from build123d import *
from OCP.BRepFilletAPI import BRepFilletAPI_MakeChamfer

# Parameters (mm, degrees)
BOSS_EXTRUDE1_DEPTH     = 15
SKETCH4_W               = 15
SKETCH4_H               = 15
BOSS_EXTRUDE2_DEPTH     = 9
CUT_EXTRUDE1_DEPTH      = 180.279015807
CUT_EXTRUDE1_DEPTH_BACK = 180.279015807
SKETCH2_R               = 2.2
SKETCH3_W               = 4.807860213
SKETCH3_H               = 184.008472667
CHAMFER1_SIZE           = 2.5
CHAMFER1_SIZE2          = 2.965251078
CHAMFER1_SIZE2_2        = 2.201823595
CHAMFER2_SIZE           = 2.5
BOSS_EXTRUDE5_DEPTH     = 3
BOSS_EXTRUDE3_DEPTH     = 2
BOSS_EXTRUDE6_DEPTH     = 2
FILLET2_R               = 1


with BuildPart() as part:
    # Sketch1 → Boss-Extrude1 (new body)
    with BuildSketch(Plane.XY):
        with BuildLine():
            Line((4.25, 16.976086121), (4.25, 10.145811944))
            ThreePointArc((4.25, 10.145811944), (0, -11), (-4.25, 10.145811944))
            Line((-4.25, 10.145811944), (-4.25, 16.976086121))
            ThreePointArc((-4.25, 16.976086121), (-12.969277239, 11.74937649), (-17.312062276, 2.557831066))
            Line((-17.312062276, 2.557831066), (-40, -151))
            Line((-40, -151), (-55, -151))
            Line((-55, -151), (-55, -160))
            Line((-55, -160), (55, -160))
            Line((55, -160), (55, -151))
            Line((55, -151), (40, -151))
            Line((40, -151), (17.312062276, 2.557831066))
            ThreePointArc((17.312062276, 2.557831066), (12.969277239, 11.74937649), (4.25, 16.976086121))
        make_face()
        Polygon((12.694157412, -17.5), (32.418580877, -151), (2.5, -151), (2.5, -17.5), align=None, mode=Mode.SUBTRACT)
        Polygon((-12.694157412, -17.5), (-2.5, -17.5), (-2.5, -151), (-32.418580877, -151), align=None, mode=Mode.SUBTRACT)
    extrude(amount=BOSS_EXTRUDE1_DEPTH)

    # Sketch4 → Boss-Extrude2 (add)
    with BuildSketch(Plane.XZ.offset(160)):
        with Locations((0, 22.5)):
            Rectangle(SKETCH4_W, SKETCH4_H)
    extrude(amount=-BOSS_EXTRUDE2_DEPTH)

    # Sketch2 → Cut-Extrude1 (cut, two sides: drawn at the far end of the back side and taken through both)
    with BuildSketch(Plane(origin=(0, -151, 0), x_dir=(1, 0, 0), z_dir=(0, 1, 0)).offset(-CUT_EXTRUDE1_DEPTH_BACK)):
        with Locations(Location((-48.75, -7.5, 0), (0, 0, 180))):
            Circle(SKETCH2_R)
        with Locations(Location((48.75, -7.5, 0), (0, 0, 270))):
            Circle(SKETCH2_R)
        with Locations(Location((0, -22.5, 0), (0, 0, 180))):
            Circle(SKETCH2_R)
    extrude(amount=CUT_EXTRUDE1_DEPTH + CUT_EXTRUDE1_DEPTH_BACK, mode=Mode.SUBTRACT)

    # Sketch3 → Cut-Revolve2 (revolve, cut)
    with BuildSketch(Plane(origin=(-48.75, 0, 0), x_dir=(0, 0, -1), z_dir=(1, 0, 0)), mode=Mode.PRIVATE) as cut_revolve2_sk:
        with Locations((-5.096069894, -58.995763666)):
            Rectangle(SKETCH3_W, SKETCH3_H)
        Polygon((-5.3, -154), (-2.692139787, -151), (-7.5, -151), (-7.5, -154), align=None)
    cut_revolve2 = revolve(cut_revolve2_sk.sketch.rotate(Axis((-48.75, -151, 7.5), (0, -1, 0)), 270), axis=Axis((-48.75, -151, 7.5), (0, -1, 0)), mode=Mode.SUBTRACT)

    # Sketch5 → Cut-Revolve3 (revolve, cut)
    with BuildSketch(Plane(origin=(0, 0, 0), x_dir=(0, 0, -1), z_dir=(1, 0, 0)), mode=Mode.PRIVATE) as cut_revolve3_sk:
        Polygon((-22.5, -151), (-22.5, -154), (-20.3, -154), (-17.692139787, -151), align=None)
    revolve(cut_revolve3_sk.sketch.rotate(Axis((0, -151, 22.5), (0, -1, 0)), 270), axis=Axis((0, -151, 22.5), (0, -1, 0)), mode=Mode.SUBTRACT)

    # Mirror1: Cut-Revolve2 across plane
    add(cut_revolve2.mirror(Plane(origin=(0, 0, 0), x_dir=(0, 0, 1), z_dir=(1, 0, 0))), mode=Mode.SUBTRACT)

    # Chamfer1: one chamfer whose edges measure the first distance from different faces: ONE call of the kernel's chamfer builder (chamfer() names one face for all edges)
    chamfer1_edges_1 = [part.edges().sort_by_distance(p)[0] for p in [
        (-2.5, -17.5, 7.5),
        (-2.5, -151, 7.5),
        (2.5, -151, 7.5),
        (2.5, -17.5, 7.5),
    ]]
    chamfer1_edges_2 = [part.edges().sort_by_distance(p)[0] for p in [
        (-12.694157412, -17.5, 7.5),
    ]]
    chamfer1_side_2 = [part.faces().sort_by_distance(p)[0] for p in [
        (-22.556369145, -84.25, 7.5),
    ]]
    chamfer1_edges_3 = [part.edges().sort_by_distance(p)[0] for p in [
        (-32.418580877, -151, 7.5),
    ]]
    chamfer1_side_3 = [part.faces().sort_by_distance(p)[0] for p in [
        (31.704168003, -151, 7.5),
    ]]
    chamfer1_edges_4 = [part.edges().sort_by_distance(p)[0] for p in [
        (32.418580877, -151, 7.5),
    ]]
    chamfer1_side_4 = [part.faces().sort_by_distance(p)[0] for p in [
        (22.556369145, -84.25, 7.5),
    ]]
    chamfer1_edges_5 = [part.edges().sort_by_distance(p)[0] for p in [
        (12.694157412, -17.5, 7.5),
    ]]
    chamfer1_side_5 = [part.faces().sort_by_distance(p)[0] for p in [
        (7.597078706, -17.5, 7.5),
    ]]
    chamfer1 = BRepFilletAPI_MakeChamfer(part.part.solid().wrapped)
    for e in chamfer1_edges_1:
        chamfer1.Add(CHAMFER1_SIZE, e.wrapped)
    for e in chamfer1_edges_2:
        chamfer1.Add(CHAMFER1_SIZE, CHAMFER1_SIZE2, e.wrapped, chamfer1_side_2[0].wrapped)  # the first distance lies on this face
    for e in chamfer1_edges_3:
        chamfer1.Add(CHAMFER1_SIZE, CHAMFER1_SIZE2_2, e.wrapped, chamfer1_side_3[0].wrapped)  # the first distance lies on this face
    for e in chamfer1_edges_4:
        chamfer1.Add(CHAMFER1_SIZE, CHAMFER1_SIZE2_2, e.wrapped, chamfer1_side_4[0].wrapped)  # the first distance lies on this face
    for e in chamfer1_edges_5:
        chamfer1.Add(CHAMFER1_SIZE, CHAMFER1_SIZE2, e.wrapped, chamfer1_side_5[0].wrapped)  # the first distance lies on this face
    add(Compound.cast(chamfer1.Shape()), mode=Mode.REPLACE)

    # Chamfer2
    chamfer2_edges = [part.edges().sort_by_distance(p)[0] for p in [
        (55, -155.5, 0),
        (-55, -155.5, 0),
        (-55, -155.5, 15),
        (55, -155.5, 15),
        (7.5, -155.5, 15),
        (7.5, -155.5, 30),
        (-7.5, -155.5, 30),
        (-7.5, -155.5, 15),
    ]]
    chamfer(chamfer2_edges, length=CHAMFER2_SIZE)

    # Sketch7 → Boss-Extrude5 (add)
    with BuildSketch(Plane.XZ.offset(160)):
        Polygon((-5, 30), (-52.5, 15), (-10, 15), (-7.5, 17.5), (-7.5, 27.5), align=None)
        Polygon((52.5, 15), (5, 30), (7.5, 27.5), (7.5, 17.5), (10, 15), align=None)
    extrude(amount=-BOSS_EXTRUDE5_DEPTH)

    # Sketch6 → Boss-Extrude3 (add)
    with BuildSketch(Plane(origin=(0, 0, 0), x_dir=(-1, 0, 0), z_dir=(0, 0, -1))):
        with BuildLine():
            Line((-4.25, 7.933315826), (-4.25, 10.145811944))
            ThreePointArc((-4.25, 10.145811944), (-6.093028803, -9.158329542), (11, 0))
            ThreePointArc((11, 0), (9.158329542, 6.093028803), (4.25, 10.145811944))
            Line((4.25, 10.145811944), (4.25, 7.933315826))
            ThreePointArc((4.25, 7.933315826), (7.721722606, 4.623310502), (9, 0))
            ThreePointArc((9, 0), (-4.623310502, -7.721722606), (-4.25, 7.933315826))
        make_face()
    extrude(amount=-BOSS_EXTRUDE3_DEPTH)

    # Sketch9 → Boss-Extrude6 (add)
    with BuildSketch(Plane.XY.offset(15)):
        with BuildLine():
            ThreePointArc((-4.25, 12.285662375), (-7.541551564, -10.588909292), (13, 0))
            ThreePointArc((13, 0), (10.588909292, 7.541551564), (4.25, 12.285662375))
            Line((4.25, 12.285662375), (4.25, 10.145811944))
            ThreePointArc((4.25, 10.145811944), (0, -11), (-4.25, 10.145811944))
            Line((-4.25, 10.145811944), (-4.25, 12.285662375))
        make_face()
    extrude(amount=BOSS_EXTRUDE6_DEPTH)

    # Fillet2
    fillet2_edges = [part.edges().sort_by_distance(p)[0] for p in [
        (-7.541551564, -10.588909292, 15),
    ]]
    fillet(fillet2_edges, radius=FILLET2_R)


solid = part.part
Here's how the part is built. I have some questions about the finished solid (model axes, mm). A direction names the side the tool comes from. Coordinates: 2 decimals unless noted, no trailing zeros. Order: outer loops, then holes, each group sorted by start corner. A loop starts at its lowest first (then second) coordinate and runs counter-clockwise, first axis right, second up. Notation, with made-up numbers: M 26.25,87.25 L 59.25,87.25 A17 ccw 59.25,110.25 Z; hole C 27,-22.5 d3. An arc over 180 degrees is marked long. Answer as CSV lines item,"result". Start each with the question number.
1. On a 3-axis mill with a long thin cutter (end or side, diameter ignored), from which of +Z, -Z, +X, -X, +Y, -Y can I reach the whole of each face in a straight line? I mean faces 1 (the flat face through (4, -11, 17)), 2 (the flat face through (-2.5, -83, 7)), 3 (the flat face through (-4.25, 13, 8)). Say none if no direction works.
2. We'd pull the mould along Z, two halves only. Please class faces 4 (the flat face through (-28.418, -158.521, 22.605)), 5 (the conical face through (46.389, -153.812, 7.396)), 6 (the cylindrical face through (46.8, -157.04, 8.52)), 7 (the flat face through (2.5, -85, 7)): released by +Z, released by -Z, zero draft, split by the parting line, or undercut.
3. I want a section at D-D, the plane z = 7.5. Count the separate pieces of the cut face and the enclosed holes in it, and give its area (3 significant figures).
4. I want a section at A-A, the plane z = 22.5. Write out the boundary of the cut face in (x, y).
5. I want a section at C-C, the plane y = -57.5. Write out the boundary of the cut face in (x, z).
6. I need wall thicknesses on line 1 (X direction, y = -34, z = 4.5); line 2 (X direction, y = -119, z = 2.5); line 3 (Z direction, x = 18, y = -44). Which ranges of each line are inside material? Lowest first, please. Write a range as [from, to].
7. For pin 1 (12 mm diameter, centred on y = -15.5, z = 5, fed in from -X); pin 2 (17.5 mm diameter, centred on x = 0, y = 0, fed in from +Z); pin 3 (7 mm diameter, centred on y = 12.5, z = 10.5, fed in from -X); pin 4 (4 mm diameter, centred on x = 23.5, y = -50, fed in from +Z), each with a flat end and sliding along its axis, tell me the tip position at first contact or that it passes through.
8. I want a section at B-B, the plane x = -22. Write out the boundary of the cut face in (y, z), and give its area (3 significant figures).
Recorded:
1,face 1,"+Z, +X, -X, +Y"
1,face 2,"+Z, -Z"
1,face 3,"+Z, -Z, +Y"
2,face 4,"released by +Z"
2,face 5,"undercut"
2,face 6,"undercut"
2,face 7,"zero draft"
3,separate pieces,"3"
3,enclosed holes,"2"
3,area,"4,320 mm2"
4,outline,"M -28.75,-160 L -2.2,-160 L -2.2,-154 L -4.81,-151 L -7.5,-151 L -7.5,-157 L -28.75,-157 Z; M 2.2,-160 L 28.75,-160 L 28.75,-157 L 7.5,-157 L 7.5,-151 L 4.81,-151 L 2.2,-154 Z"
5,outline,"M -26.19,0 L -18.6,0 L -18.6,15 L -26.19,15 Z; M -2.5,0 L 2.5,0 L 2.5,15 L -2.5,15 Z; M 18.6,0 L 26.19,0 L 26.19,15 L 18.6,15 Z"
6,line 1,"x = [-22.71, -15.13], [-2.5, 2.5], [15.13, 22.71]"
6,line 2,"x = [-35.27, -27.69], [-2.5, 2.5], [27.69, 35.27]"
6,line 3,"z = [0, 15]"
7,pin 1,"stops at x = -20.87"
7,pin 2,"passes through"
7,pin 3,"stops at x = -15.01"
7,pin 4,"stops at z = 15"
8,outline,"M -160,0 L -151,0 L -151,15 L -157,15 L -157,24.63 L -160,24.63 Z; M -80.48,0 L -29.17,0 L -29.17,15 L -80.48,15 Z"
8,area,"934 mm2"
